Study the drawing (mm; zero at the part's minimum x, y, z) and answer. A direction names the side the tool comes from. Give positions to 0.01 mm unless a question says otherwise; leave off trailing zeros. Write each loop counter-clockwise with the first axis right and the second up, starting at its lowest first coordinate (ties: lowest second). Pieces come first, ordered by that corner, then holes. Notation, with made-up numbers: M 51.5,65 L 110.5,65 A17 ccw 110.5,86 Z; hole C -13,22 d6. An arc over 180 degrees is marked long. Use a Markdown table: item, result. Add a question column.
Item 1: For the marked faces 1, 2, 3, 4 and 5, determine the directions among +Z, -Z, +X, -X, +Y, -Y from which every point of the face is accessible in a straight line to the end or side of a thin tool.
Item 2: A cutting plane is placed at A-A on y = 81. Count the separate pieces of the cut face and the enclosed holes in it, then the cut area to 3 significant figures.
Item 3: The mould has two halves that part along X. Classify the marked faces 6, 7, 8 and 9: pulls with the +X half, pulls with the -X half, needs draft (parallel to the pull), parting line crosses it, or undercut.
Item 4: A cutting plane is placed at C-C on x = 103. Determine the outline of the cut face in (y, z).
Item 5: Consider probe 1 along Y at (x, z) = (92, 66.5); probe 2 along X at (y, z) = (95.5, 82) (1 decimal); probe 3 along X at (y, z) = (52, 133). Determine where each line is inside the solid, lowest interval first. Write a range as [from, to].
Item 6: A cutting plane is placed at B-B on z = 93. Determine the outline of the cut face in (x, y).
Item 7: Given P1, Ø1, axis at y = 33, z = 120, coming from the +X side; P2, Ø17, axis at x = 142.5, y = 63.5, coming from the -Z side; P3, Ø4, axis at y = 37.5, z = 134, coming from the +X side; P4, Ø17, axis at y = 64, z = 129, coming from the -X side, each flat-ended and moving along its own axis, determine where each tip first touches the part or whether it passes through.
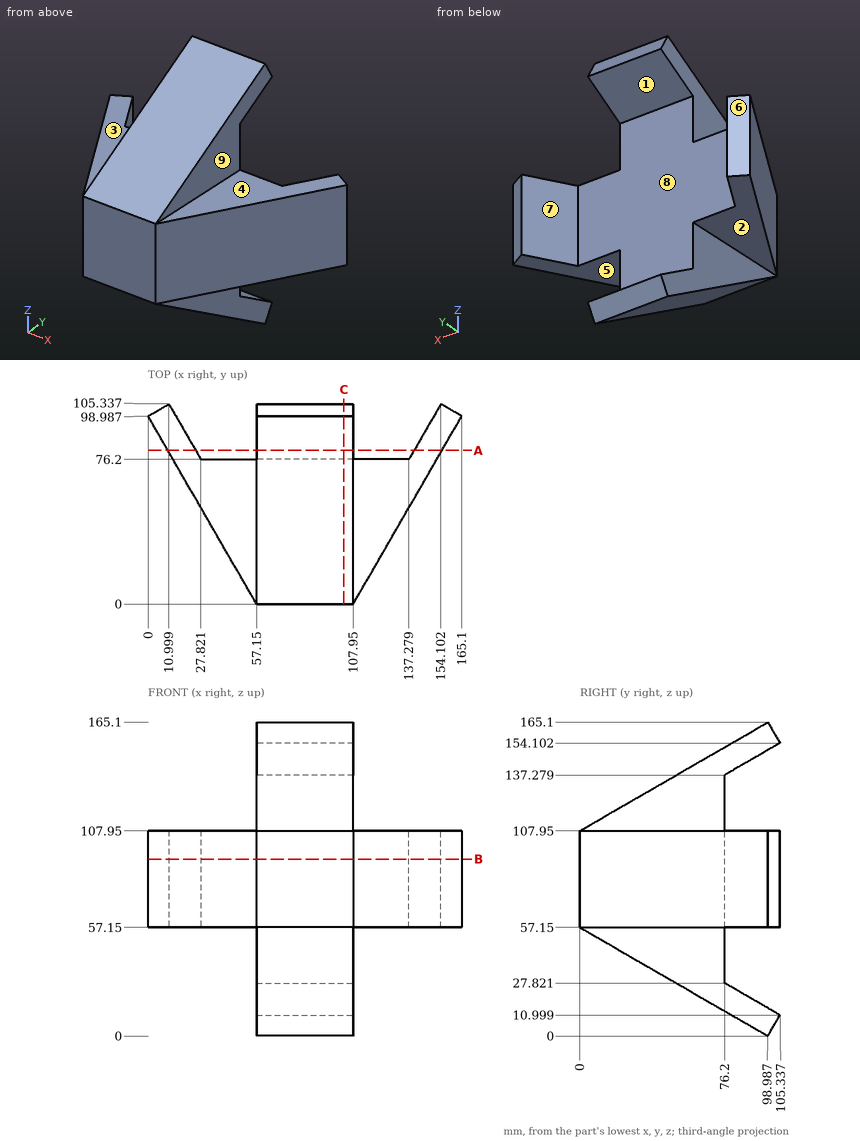
Filled in:
| question | item | result |
|---|---|---|
| 1 | face 1 | +X, -X, +Y |
| 1 | face 2 | -Z, -X, +Y, -Y |
| 1 | face 3 | +Z, -X, +Y, -Y |
| 1 | face 4 | +Z, +X, +Y, -Y |
| 1 | face 5 | -Z, +X, +Y, -Y |
| 2 | separate pieces | 4 |
| 2 | enclosed holes | 0 |
| 2 | area | 2,980 mm² |
| 3 | face 6 | pulls with the -X half |
| 3 | face 7 | undercut |
| 3 | face 8 | undercut |
| 3 | face 9 | pulls with the +X half |
| 4 | outline | M 0,57.15 L 98.99,0 L 105.34,11 L 76.2,27.82 L 76.2,137.28 L 105.34,154.1 L 98.99,165.1 L 0,107.95 Z |
| 5 | probe 1 | [0, 76.2] |
| 5 | probe 2 | [2, 16.7], [148.4, 163.1] |
| 5 | probe 3 | [57.15, 107.95] |
| 6 | outline | M 0,98.99 L 57.15,0 L 107.95,0 L 165.1,98.99 L 154.1,105.34 L 137.28,76.2 L 27.82,76.2 L 11,105.34 Z |
| 7 | P1 | x = 107.95 |
| 7 | P2 | z = 57.15 |
| 7 | P3 | through |
| 7 | P4 | x = 57.15 |
